The model under review builds one solid part; all positions refer to its coordinate system, in mm. Face numbers are marked on the shaded views. A direction names the side the tool comes from. Round coordinates to 2 decimals unless told otherwise and drop trailing zeros. Loops run counter-clockwise (first coordinate to the right, second up) from the corner with the lowest first, then second, coordinate; pieces in that order, holes last. Notation, with made-up numbers: (-29.5, 74) -> (5.5, 74) arc R6 cw to (5.5, 79) -> close; hole circle Ø4 at (-7.5, -32.5). An arc over 180 degrees is marked (long way). Use a Markdown table: item, result. Add a question column.
1) Consider section C-C on z = 2.25. Give the boundary of the cut face in (x, y).
2) Consider section D-D on x = 2.25. Give the boundary of the cut face in (y, z).
3) Insertion check: pin 1 (1.5 mm diameter, centred on x = 8, y = -1.5, fed in from +Z); pin 2 (2 mm diameter, centred on y = -3, z = 6.5, fed in from +X); pin 3 (0.6 mm diameter, centred on x = -5.5, z = 0.5, fed in from -Y). Each pin has a flat end and moves straight along its axis. Give the tip position at first contact, or say it passes through.
4) Mouldability with a two-part tool opening along X and no side actions: class the marked faces 1, 2 and 3 as released by +X, released by -X, zero draft, split by the parting line, or undercut.
5) Wall thickness on probe 1 along Z at (x, y) = (-13.7, 0); probe 2 along X at (y, z) = (0.25, 9.25); probe 3 along Z at (x, y) = (-9.5, -2): over which ranges is each line inside the solid? List them lowest first.
6) For the marked faces 4, 5 and 6, list the 3-axis set-ups (+Z, -Z, +X, -X, +Y, -Y) from which the entire face can be reached by the end or side of a thin tool; tool diameter is ignored.
7) Consider section B-B on z = 7.5. Give the boundary of the cut face in (x, y).
8) Consider section A-A on x = -8.5. Give the boundary of the cut face in (y, z).
from build123d import *

# Parameters (mm, degrees)
F0_R     = 1.27
F1_DEPTH = 1.27
F2_W     = 5.08
F2_H     = 11.43
F3_DEPTH = 8.89
F4_R     = 3.302
F5_DEPTH = 21.336
F6_R     = 1.27


with BuildPart() as f1:
    # F0 (on Top) → F1 (new body)
    with BuildSketch(Plane.XY):
        with BuildLine():
            Line((-10.668, 5.715), (-15.748, 5.715))
            Line((-15.748, 5.715), (-15.748, -5.715))
            Line((-15.748, -5.715), (-10.668, -5.715))
            Line((-10.668, -5.715), (-10.668, -2.54))
            Line((-10.668, -2.54), (0.508, -2.54))
            Line((0.508, -2.54), (0.508, -5.715))
            Line((0.508, -5.715), (5.588, -5.715))
            Line((5.588, -5.715), (5.588, -2.54))
            Line((5.588, -2.54), (8.128, -2.54))
            ThreePointArc((8.128, -2.54), (10.668, 0), (8.128, 2.54))
            Line((8.128, 2.54), (5.588, 2.54))
            Line((5.588, 2.54), (5.588, 5.715))
            Line((5.588, 5.715), (0.508, 5.715))
            Line((0.508, 5.715), (0.508, 2.54))
            Line((0.508, 2.54), (-10.668, 2.54))
            Line((-10.668, 2.54), (-10.668, 5.715))
        make_face()
        with Locations((-8.128, 0)):
            Circle(F0_R, mode=Mode.SUBTRACT)
        with Locations((8.128, 0)):
            Circle(F0_R, mode=Mode.SUBTRACT)
    extrude(amount=F1_DEPTH)

    # F2 (on face) → F3 (join)
    with BuildSketch(Plane.XY.offset(1.27)):
        with Locations((-13.208, 0)):
            Rectangle(F2_W, F2_H)
        with Locations((3.048, 0)):
            Rectangle(F2_W, F2_H)
    extrude(amount=F3_DEPTH)

    # F4 (on face) → F5 (cut, through all)
    with BuildSketch(Plane.YZ.offset(5.588)):
        with Locations((0, 5.842)):
            Circle(F4_R)
        with BuildLine():
            Line((5.715, 10.16), (0, 10.16))
            ThreePointArc((0, 10.16), (3.053287, 8.895287), (4.318, 5.842))
            Line((4.318, 5.842), (4.318, 0))
            Line((4.318, 0), (5.715, 0))
            Line((5.715, 0), (5.715, 10.16))
        make_face()
        with BuildLine():
            Line((-5.715, 0), (-4.318, 0))
            Line((-4.318, 0), (-4.318, 5.842))
            ThreePointArc((-4.318, 5.842), (-3.053287, 8.895287), (0, 10.16))
            Line((0, 10.16), (-5.715, 10.16))
            Line((-5.715, 10.16), (-5.715, 0))
        make_face()
    extrude(amount=-F5_DEPTH, mode=Mode.SUBTRACT)

    # F6
    f6_edges = [f1.edges().sort_by_distance(p)[0] for p in [
        (-10.668, -2.54, 0.635),
        (5.588, -2.54, 0.635),
        (0.508, -2.54, 0.635),
        (0.508, 2.54, 0.635),
        (5.588, 2.54, 0.635),
        (-10.668, 2.54, 0.635),
    ]]
    fillet(f6_edges, radius=F6_R)


solid = f1.part
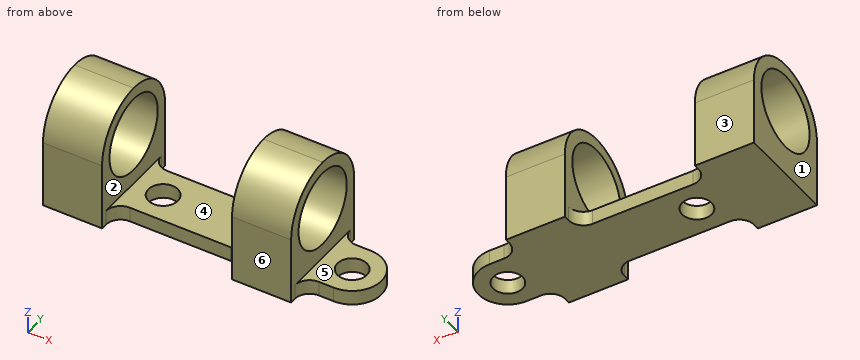
Result set:
| question | item | result |
|---|---|---|
| 1 | outline | (-15.75, -4.32) -> (-10.67, -4.32) -> (-10.67, 4.32) -> (-15.75, 4.32) -> close; (0.51, -4.32) -> (5.59, -4.32) -> (5.59, 4.32) -> (0.51, 4.32) -> close |
| 2 | outline | (-4.32, 0) -> (4.32, 0) -> (4.32, 5.84) arc R4.32 ccw to (-4.32, 5.84) -> close; hole circle Ø6.6 at (0, 5.84) |
| 3 | pin 1 | z = 1.27 |
| 3 | pin 2 | x = 5.59 |
| 3 | pin 3 | y = -2.54 |
| 4 | face 1 | released by -X |
| 4 | face 2 | undercut |
| 4 | face 3 | zero draft |
| 5 | probe 1 | 0 to 2.54, 9.14 to 10.16 |
| 5 | probe 2 | -15.75 to -10.67, 0.51 to 5.59 |
| 5 | probe 3 | 0 to 1.27 |
| 6 | face 4 | +Z, +Y, -Y |
| 6 | face 5 | +Z, +X, +Y, -Y |
| 6 | face 6 | +Z, -Z, +X, -X, -Y |
| 7 | outline | (-15.75, -3.99) -> (-10.67, -3.99) -> (-10.67, -2.86) -> (-15.75, -2.86) -> close; (-15.75, 2.86) -> (-10.67, 2.86) -> (-10.67, 3.99) -> (-15.75, 3.99) -> close; (0.51, -3.99) -> (5.59, -3.99) -> (5.59, -2.86) -> (0.51, -2.86) -> close; (0.51, 2.86) -> (5.59, 2.86) -> (5.59, 3.99) -> (0.51, 3.99) -> close |
| 8 | outline | (-2.54, 0) -> (-1.21, 0) -> (-1.21, 1.27) -> (-2.54, 1.27) -> close; (1.21, 0) -> (2.54, 0) -> (2.54, 1.27) -> (1.21, 1.27) -> close |
